Verification items for the finished model (mm, model axes). Give positions to 0.01 mm unless a question says otherwise; leave off trailing zeros. Loops run counter-clockwise (first coordinate to the right, second up) from the corner with the lowest first, then second, coordinate; pieces in that order, holes last. Notation, with made-up numbers: (39.5, -19.75) - (62.5, -19.75) arc R19 cw to (62.5, -5.75) - close; hole circle Ø5 at (84.5, 87.5). An arc over 180 degrees is marked (long way). One line per item, written item: value. Start each with the question number.
1. Sectioned sample at C-C (x = 76.2). Record the cut outline in (y, z) (3 decimals).
2. Sectioned sample at A-A (y = 25.4). Record the cut outline in (x, z) (3 decimals).
3. Scan lines: L1, parallel to X at y = 76.2, z = 2; L2, parallel to Y at x = 127, z = 2.75. Record each from-to range of solid material in increasing order. Write a range as [from, to].
4. Sectioned sample at D-D (z = 1.5). Record the cut outline in (x, y).
5. Gauge pin test, flat end, axial feed: pin 1 (10.5 mm diameter, centred on x = 25.4, y = 76.2, fed in from +Z) (3 decimals). Record the tip position at first contact, or that the pin passes through.
from build123d import *

# Parameters (mm, degrees)
SKETCH1_W             = 152.4
SKETCH1_H             = 152.4
PLATE_DEPTH           = 9.525
SKETCH3_R             = 3.96875
BOLT_ONE_SKETCH_DEPTH = 216.736518988
SKETCH4_R             = 12.7
CENTRE_BORE2_DEPTH    = 216.736518988


with BuildPart() as part:
    # Sketch1 → plate (new body)
    with BuildSketch(Plane.XY):
        with Locations((76.2, 76.2)):
            Rectangle(SKETCH1_W, SKETCH1_H)
    extrude(amount=PLATE_DEPTH)

    # Sketch3 → bolt_one_sketch (cut, through all)
    with BuildSketch(Plane.XY):
        with Locations((127, 76.2)):
            Circle(SKETCH3_R)
        with Locations((76.2, 127)):
            Circle(SKETCH3_R)
        with Locations((25.4, 76.2)):
            Circle(SKETCH3_R)
        with Locations((76.2, 25.4)):
            Circle(SKETCH3_R)
    extrude(amount=BOLT_ONE_SKETCH_DEPTH, mode=Mode.SUBTRACT)

    # Sketch4 → centre_bore2 (cut, through all)
    with BuildSketch(Plane.XY):
        with Locations((76.2, 76.2)):
            Circle(SKETCH4_R)
    extrude(amount=CENTRE_BORE2_DEPTH, mode=Mode.SUBTRACT)


solid = part.part
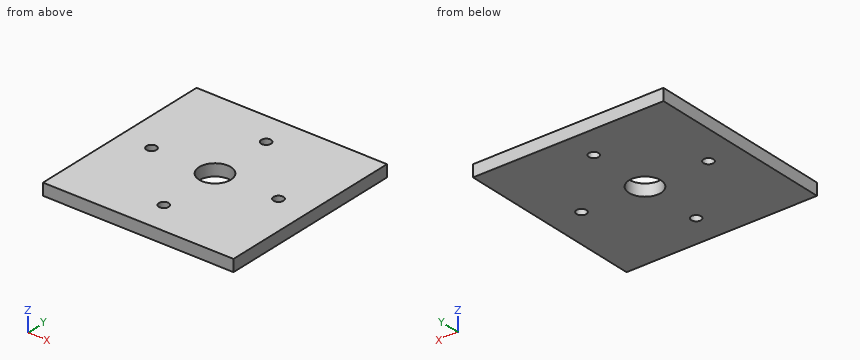
Results are:
1. outline: (0, 0) - (21.431, 0) - (21.431, 9.525) - (0, 9.525) - close; (29.369, 0) - (63.5, 0) - (63.5, 9.525) - (29.369, 9.525) - close; (88.9, 0) - (123.031, 0) - (123.031, 9.525) - (88.9, 9.525) - close; (130.969, 0) - (152.4, 0) - (152.4, 9.525) - (130.969, 9.525) - close
2. outline: (0, 0) - (72.231, 0) - (72.231, 9.525) - (0, 9.525) - close; (80.169, 0) - (152.4, 0) - (152.4, 9.525) - (80.169, 9.525) - close
3. L1: x = [0, 21.43], [29.37, 63.5], [88.9, 123.03], [130.97, 152.4]
3. L2: y = [0, 72.23], [80.17, 152.4]
4. outline: (0, 0) - (152.4, 0) - (152.4, 152.4) - (0, 152.4) - close; hole circle Ø7.94 at (25.4, 76.2); hole circle Ø25.4 at (76.2, 76.2); hole circle Ø7.94 at (76.2, 25.4); hole circle Ø7.94 at (76.2, 127); hole circle Ø7.94 at (127, 76.2)
5. pin 1: stops at z = 9.525
